```python
from build123d import *

# Parameters (mm, degrees)
F0_R     = 3.175
F0_R_2   = 11
F1_DEPTH = 3
F3_R     = 5
F5_DEPTH = 6


with BuildPart() as f1:
    # F0 (on Front) → F1 (new body)
    with BuildSketch(Plane.XZ):
        with BuildLine():
            Line((35, 35), (-15, 35))
            Line((-15, 35), (-15, -35))
            Line((-15, -35), (35, -35))
            ThreePointArc((35, -35), (70, 0), (35, 35))
        make_face()
        with Locations((0, -19)):
            Circle(F0_R, mode=Mode.SUBTRACT)
        with Locations((0, 19)):
            Circle(F0_R, mode=Mode.SUBTRACT)
        with Locations((35, 0)):
            Circle(F0_R_2, mode=Mode.SUBTRACT)
    extrude(amount=F1_DEPTH)

    # F2: F1 across plane


with BuildPart() as f1_1:
    add(f1.part)
    add(f1.part.mirror(Plane.XY))

    # F3
    f3_edges = [f1_1.edges().sort_by_distance(p)[0] for p in [
        (-15, -1.5, -35),
        (-15, -1.5, 35),
    ]]
    fillet(f3_edges, radius=F3_R)

    # F4 (on face) → F5 (join)
    with BuildSketch(Plane(origin=(0, 0, 0), x_dir=(-1, 0, 0), z_dir=(0, 1, 0))):
        with BuildLine():
            Line((-35, -35), (10, -35))
            ThreePointArc((10, -35), (13.5355339059, -33.5355339059), (15, -30))
            Line((15, -30), (15, 30))
            ThreePointArc((15, 30), (13.5355339059, 33.5355339059), (10, 35))
            Line((10, 35), (-35, 35))
            ThreePointArc((-35, 35), (-70, 0), (-35, -35))
        make_face()
        with BuildLine():
            Line((-35, 31), (11, 31))
            Line((11, 31), (11, -31))
            Line((11, -31), (-35, -31))
            ThreePointArc((-35, -31), (-66, 0), (-35, 31))
        make_face(mode=Mode.SUBTRACT)
    extrude(amount=F5_DEPTH)


solid = f1_1.part
```
For this review, take the finished solid that the model builds, in its own axes (mm). A direction names the side the tool comes from. Coordinates: 2 decimals unless noted, no trailing zeros. Order: outer loops, then holes, each group sorted by start corner. A loop starts at its lowest first (then second) coordinate and runs counter-clockwise, first axis right, second up. Notation, with made-up numbers: (73.25, 22) -> (87.25, 22) arc R9 cw to (87.25, 28) -> close; hole circle Ø3 at (21, 19). An arc over 180 degrees is marked (long way). Use CSV: the item, a comma, the result in double quotes. Start each with the question number.
Item 1: We need section D-D, the plane x = 63.5. Give the boundary of the cut face in (y, z).
Item 2: We need section A-A, the plane y = 1. Give the boundary of the cut face in (x, z), then the cut area to 3 significant figures.
Item 3: Wall thickness on probe 1 along Z at (x, y) = (0, -1.2) (3 decimals); probe 2 along Z at (x, y) = (35, -2.2); probe 3 along Z at (x, y) = (24.5, 1.5): over which ranges is each line inside the solid? List them lowest first.
Item 4: We need section C-C, the plane x = 44. Give the boundary of the cut face in (y, z), then the cut area to 3 significant figures.
Item 5: Draft analysis for pull direction X (two halves, no side actions). For faces 3 (the face through (69.99, 1.44, 0.77)), 4 (the face through (18, 0, 0)), 5 (the face through (12, 1, 35)), 6 (the face through (12, 3, 31)), state which applies: pulls with the +X half, pulls with the -X half, needs draft (parallel to the pull), parting line crosses it, or undercut.
Item 6: Insertion check: pin 1 (4 mm diameter, centred on y = 4, z = 19, fed in from +X); pin 2 (3 mm diameter, centred on y = 3, z = -3, fed in from +X); pin 3 (8.5 mm diameter, centred on x = 0, z = -19, fed in from +Y). Each pin has a flat end and moves straight along its axis. Give the tip position at first contact, or say it passes through.
Item 7: For faces 1 (the face through (13, 1, -35)), 2 (the face through (65.993, 2.958, -0.682)), list the 3-axis set-ups (+Z, -Z, +X, -X, +Y, -Y) from which the entire face can be reached by the end or side of a thin tool; tool diameter is ignored.
Item 8: We need section B-B, the plane z = 0. Give the boundary of the cut face in (x, y).
Derived:
1,outline,"(-3, -20.32) -> (6, -20.32) -> (6, -12.2) -> (0, -12.2) -> (0, 12.2) -> (6, 12.2) -> (6, 20.32) -> (-3, 20.32) -> close"
2,outline,"(-15, -30) arc R5 ccw to (-10, -35) -> (35, -35) arc R35 ccw to (35, 35) -> (-10, 35) arc R5 ccw to (-15, 30) -> close; hole (-11, -31) -> (35, -31) arc R31 ccw to (35, 31) -> (-11, 31) -> close"
2,area,"1,050 mm^2"
3,probe 1,"z = -35 to -22.175, -15.825 to 15.825, 22.175 to 35"
3,probe 2,"z = -35 to -11, 11 to 35"
3,probe 3,"z = -35 to -31, 31 to 35"
4,outline,"(-3, -33.82) -> (6, -33.82) -> (6, -29.66) -> (0, -29.66) -> (0, -6.32) -> (-3, -6.32) -> close; (-3, 6.32) -> (0, 6.32) -> (0, 29.66) -> (6, 29.66) -> (6, 33.82) -> (-3, 33.82) -> close"
4,area,"215 mm^2"
5,face 3,"pulls with the +X half"
5,face 4,"undercut"
5,face 5,"needs draft"
5,face 6,"undercut"
6,pin 1,"stops at x = 65.59"
6,pin 2,"stops at x = 69.97"
6,pin 3,"stops at y = 0"
7,face 1,"-Z, +X, -X, +Y, -Y"
7,face 2,"+Y"
8,outline,"(-15, -3) -> (24, -3) -> (24, 0) -> (-11, 0) -> (-11, 6) -> (-15, 6) -> close; (46, -3) -> (70, -3) -> (70, 6) -> (66, 6) -> (66, 0) -> (46, 0) -> close"
